Read the model definition and answer for the solid it produces. Units are mm, in the model's axes. A direction names the side the tool comes from. Coordinates: 2 decimals unless noted, no trailing zeros. Write each loop counter-clockwise with the first axis right and the second up, starting at its lowest first coordinate (ties: lowest second). Pieces come first, ordered by that corner, then holes. Notation, with made-up numbers: M 17,-27.5 L 41,-27.5 A21 cw 41,-0.5 Z; hole C -21,-37.5 d6. An arc over 180 degrees is marked long. Use a Markdown table: item, result. Add a question column.
from build123d import *

# Parameters (mm, degrees)
SKETCH1_W           = 104.902
SKETCH1_H           = 48.26
BOSS_EXTRUDE1_DEPTH = 1.27
SKETCH1_3_W         = 104.902
SKETCH1_3_H         = 1.27
BOSS_EXTRUDE2_DEPTH = 38.1
CUT_EXTRUDE1_DEPTH  = 53.34


with BuildPart() as part:
    # Sketch1 → Boss-Extrude1 (new body)
    with BuildSketch(Plane(origin=(0, 0, 0), x_dir=(1, 0, 0), z_dir=(0, 1, 0))):
        with Locations((3.8862, -0.511112371)):
            Rectangle(SKETCH1_W, SKETCH1_H)
    extrude(amount=BOSS_EXTRUDE1_DEPTH)

    # Sketch1<3> → Boss-Extrude2 (add)
    with BuildSketch(Plane(origin=(0, 0, 0), x_dir=(1, 0, 0), z_dir=(0, 1, 0))):
        with Locations((3.8862, -25.276112371)):
            Rectangle(SKETCH1_3_W, SKETCH1_3_H)
        with Locations((3.8862, 24.253887629)):
            Rectangle(SKETCH1_3_W, SKETCH1_3_H)
    extrude(amount=BOSS_EXTRUDE2_DEPTH)

    # Sketch2 → Cut-Extrude1 (cut)
    with BuildSketch(Plane.XY.offset(25.911112371)):
        Polygon((-48.5648, 15.307256031), (44.262468269, 38.1), (-48.5648, 38.1), align=None)
    extrude(amount=-CUT_EXTRUDE1_DEPTH, mode=Mode.SUBTRACT)


solid = part.part
Item 1: Find section C-C on z = -6. Give the vertices of the cut face in (x, y).
Item 2: Consider probe 1 along Z at (x, y) = (-2, 19.5); probe 2 along Y at (x, z) = (-43, -1). Determine where each line is inside the solid, lowest interval first.
Item 3: Find section D-D on y = 30.5. Give the vertices of the cut face in (x, z), then the cut area to 3 significant figures.
Item 4: Find section A-A on y = 6.5. Give the vertices of the cut face in (x, z).
Item 5: Find section B-B on x = 6. Give the vertices of the cut face in (y, z).
Item 6: This flat-tipped pin is pushed along its axis until it touches: pin 1 (24 mm diameter, centred on x = 17.5, z = -0.5, fed in from +Y). Where does it stop, or does it pass through?
Item 7: Determine the mould class of faces 3 (the flat face through (15, 15, -23.619)), 4 (the flat face through (3, 0, 0)), 5 (the flat face through (15, 15, -24.889)) for opening direction Z: pulls with the +Z half, pulls with the -Z half, needs draft (parallel to the pull), parting line crosses it, or undercut.
Item 8: For faces 1 (the flat face through (15, 15, 24.641)), 2 (the flat face through (-48.565, 1, 3)), determine the directions among +Z, -Z, +X, -X, +Y, -Y from which every point of the face is accessible in a straight line to the end or side of a thin tool.
Geometry says:
| question | item | result |
|---|---|---|
| 1 | outline | M -48.56,0 L 56.34,0 L 56.34,1.27 L -48.56,1.27 Z |
| 2 | probe 1 | z = -24.89 to -23.62, 24.64 to 25.91 |
| 2 | probe 2 | y = 0 to 1.27 |
| 3 | outline | M 13.31,-24.89 L 56.34,-24.89 L 56.34,-23.62 L 13.31,-23.62 Z; M 13.31,24.64 L 56.34,24.64 L 56.34,25.91 L 13.31,25.91 Z |
| 3 | area | 109 mm2 |
| 4 | outline | M -48.56,-24.89 L 56.34,-24.89 L 56.34,-23.62 L -48.56,-23.62 Z; M -48.56,24.64 L 56.34,24.64 L 56.34,25.91 L -48.56,25.91 Z |
| 5 | outline | M 0,-24.89 L 28.71,-24.89 L 28.71,-23.62 L 1.27,-23.62 L 1.27,24.64 L 28.71,24.64 L 28.71,25.91 L 0,25.91 Z |
| 6 | pin 1 | stops at y = 1.27 |
| 7 | face 3 | undercut |
| 7 | face 4 | needs draft |
| 7 | face 5 | pulls with the -Z half |
| 8 | face 1 | +X, -X, +Y |
| 8 | face 2 | +Z, -Z, -X, +Y, -Y |
